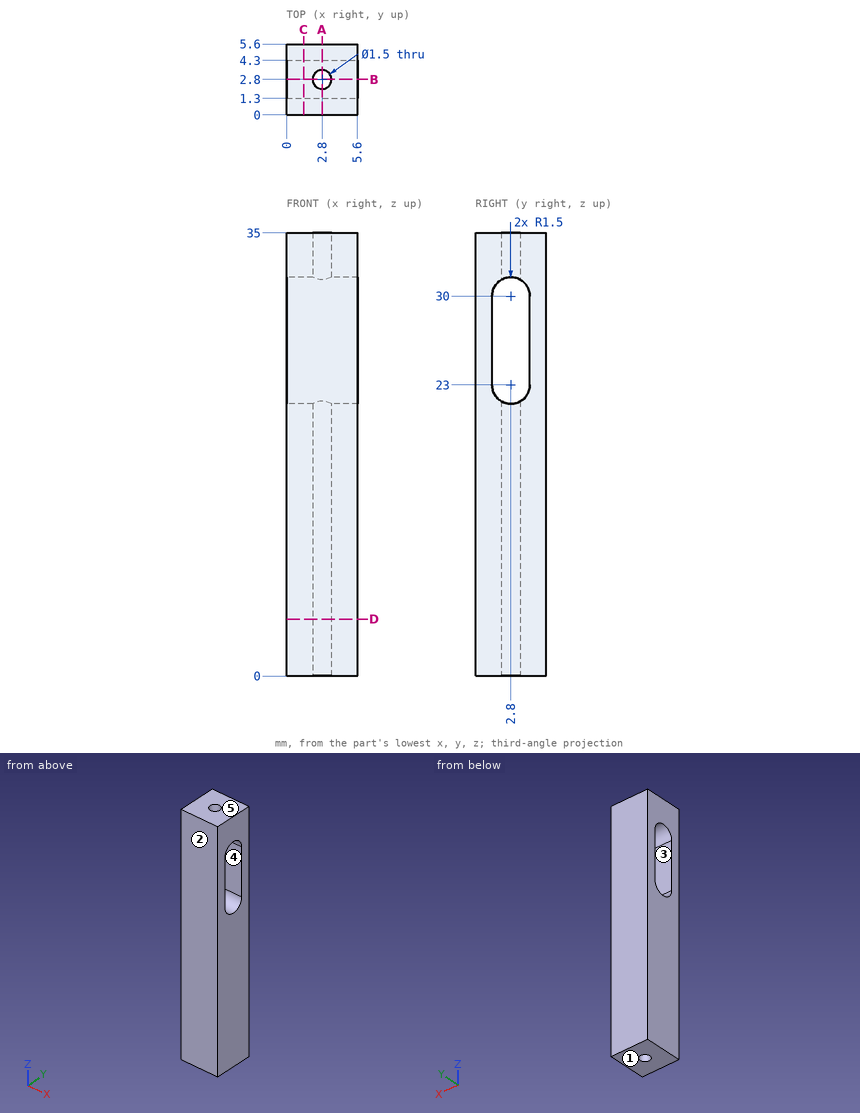
For this review, use the dimensioned drawing (mm, ordinates from the lowest corner) and the shaded views. A direction names the side the tool comes from. Round coordinates to 2 decimals unless told otherwise and drop trailing zeros. Order: outer loops, then holes, each group sorted by start corner. A loop starts at its lowest first (then second) coordinate and runs counter-clockwise, first axis right, second up. Notation, with made-up numbers: (-38, -33.75) - (13, -33.75) arc R28 ccw to (13, 3.25) - close; hole circle Ø7 at (-37.75, 62). An arc over 180 degrees is marked (long way). Use one line per item in the form item = value.
Q1. Add section D-D on z = 4.5. Give the boundary of the cut face in (x, y), then the cut area to 3 significant figures.
Response values:
outline = (0, 0) - (5.6, 0) - (5.6, 5.6) - (0, 5.6) - close; hole circle Ø1.5 at (2.8, 2.8)
area = 29.6 mm^2
Q2. Add section C-C on x = 1.35. Give the boundary of the cut face in (y, z), then the cut area to 3 significant figures.
Response values:
outline = (0, 0) - (5.6, 0) - (5.6, 35) - (0, 35) - close; hole (1.3, 23) arc R1.5 ccw to (4.3, 23) - (4.3, 30) arc R1.5 ccw to (1.3, 30) - close
area = 168 mm^2
Q3. Add section A-A on x = 2.8. Give the boundary of the cut face in (y, z), then the cut area to 3 significant figures.
Response values:
outline = (0, 0) - (2.05, 0) - (2.05, 21.7) arc R1.5 cw to (1.3, 23) - (1.3, 30) arc R1.5 cw to (2.05, 31.3) - (2.05, 35) - (0, 35) - close; (3.55, 0) - (5.6, 0) - (5.6, 35) - (3.55, 35) - (3.55, 31.3) arc R1.5 cw to (4.3, 30) - (4.3, 23) arc R1.5 cw to (3.55, 21.7) - close
area = 130 mm^2
Q4. Clearance check with a flat-ended pin moving along its axis: P1, Ø2, axis at x = 2.8, y = 2.8, coming from the +Z side. State where the tip first meets the part, or that it passes through.
Response values:
P1 = 35
Q5. Add section B-B on y = 2.8. Give the boundary of the cut face in (x, z), then the cut area to 4 significant figures.
Response values:
outline = (0, 0) - (2.05, 0) - (2.05, 21.5) - (0, 21.5) - close; (0, 31.5) - (2.05, 31.5) - (2.05, 35) - (0, 35) - close; (3.55, 0) - (5.6, 0) - (5.6, 21.5) - (3.55, 21.5) - close; (3.55, 31.5) - (5.6, 31.5) - (5.6, 35) - (3.55, 35) - close
area = 102.5 mm^2
Q6. Tool access review of the marked faces 4 and 5: name each direction out of +Z, -Z, +X, -X, +Y, -Y from which nothing blocks a thin tool from reaching the whole face with its end or side.
Response values:
face_4 = +X, -X
face_5 = +Z, +X, -X, +Y, -Y
Q7. Mouldability with a two-part tool opening along Y and no side actions: class the marked faces 1, 2 and 3 as pulls with the +Y half, pulls with the -Y half, needs draft (parallel to the pull), parting line crosses it, or undercut.
Response values:
face_1 = needs draft
face_2 = pulls with the -Y half
face_3 = undercut
Q8. To check wall thickness, follow line 1 (X direction, y = 2.8, z = 33.7); line 2 (Y direction, x = 1.25, z = 26). State the ranges of each line that lie inside material, in increasing order.
Response values:
line_1 = 0 to 2.05, 3.55 to 5.6
line_2 = 0 to 1.3, 4.3 to 5.6
